Input: part model. Units: mm. Frame: model coordinates. Face numbers are marked on the shaded views. Give positions to 0.01 mm unless a question says otherwise; leave off trailing zeros. Write each loop counter-clockwise with the first axis right and the second up, starting at its lowest first coordinate (ties: lowest second). Pieces come first, ordered by that corner, then holes. Notation, with made-up numbers: (83, 37) - (91, 37) arc R35 cw to (91, 76) - close; hole circle Ø1 at (59, 31.25). An arc over 180 degrees is marked (long way). Use a Markdown table: item, result. Add a question column.
1. Section query D-D, the plane y = 10. Return loops of the section in (x, z), plus the area to 3 significant figures.
2. Section query C-C, the plane y = 3.75. Return loops of the section in (x, z), plus the area to 3 significant figures.
3. Section query B-B, the plane x = 70. Return loops of the section in (y, z).
4. Section query A-A, the plane z = 10.5. Return loops of the section in (x, y).
5. Mould query, pull axis Y, two halves, no side actions, for the marked faces 1, 2, 3 and 4. Classes: released by +Y, released by -Y, zero draft, split by the parting line, or undercut.
6. Pin query (flat end, axial travel): pin 1 (2 mm diameter, centred on y = -2, z = 11.5, fed in from -X). Return the tip coordinate at first contact, or that it passes through.
7. Material intervals for probe 1 along Y at (x, z) = (75, 12.5); probe 2 along X at (y, z) = (-2, 2.5); probe 3 along X at (y, z) = (4.25, 8.75), sorted ascending.
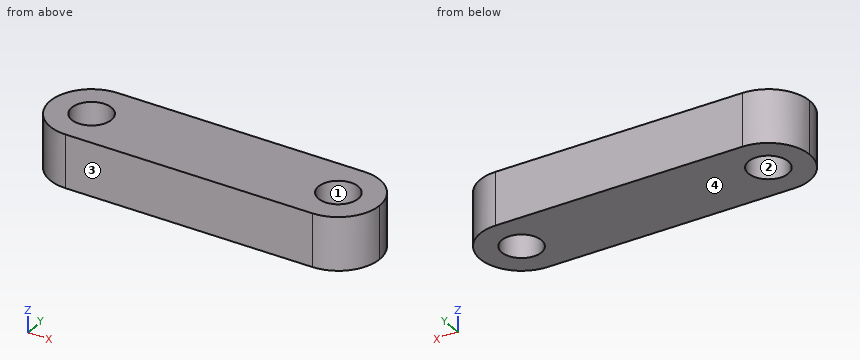
```python
from build123d import *

# Parameters (mm, degrees)
F0_R     = 6
F1_DEPTH = 16


# Not quite as in the source:
# - a feature names something its author has since deleted; it is built from what else it names


with BuildPart() as f1:
    # F0 (on Top) → F1 (new body)
    with BuildSketch(Plane.XY):
        with BuildLine():
            Line((75, 12.5), (0, 12.5))
            ThreePointArc((0, 12.5), (8.8388347648, 8.8388347648), (12.5, 0))
            ThreePointArc((12.5, 0), (8.8388347648, -8.8388347648), (0, -12.5))
            Line((0, -12.5), (75, -12.5))
            ThreePointArc((75, -12.5), (62.5, 0), (75, 12.5))
        make_face()
        with BuildLine():
            ThreePointArc((12.5, 0), (8.8388347648, 8.8388347648), (0, 12.5))
            ThreePointArc((0, 12.5), (-8.8388347648, 8.8388347648), (-12.5, 0))
            ThreePointArc((-12.5, 0), (-8.8388347648, -8.8388347648), (0, -12.5))
            ThreePointArc((0, -12.5), (8.8388347648, -8.8388347648), (12.5, 0))
        make_face()
        Circle(F0_R, mode=Mode.SUBTRACT)
        with BuildLine():
            ThreePointArc((87.5, 0), (83.8388347648, 8.8388347648), (75, 12.5))
            ThreePointArc((75, 12.5), (62.5, 0), (75, -12.5))
            ThreePointArc((75, -12.5), (83.8388347648, -8.8388347648), (87.5, 0))
        make_face()
        with Locations((75, 0)):
            Circle(F0_R, mode=Mode.SUBTRACT)
    extrude(amount=F1_DEPTH)


solid = f1.part
```
Result sheet:
| question | item | result |
|---|---|---|
| 1 | outline | (-7.5, 0) - (82.5, 0) - (82.5, 16) - (-7.5, 16) - close |
| 1 | area | 1,440 mm² |
| 2 | outline | (-11.92, 0) - (-4.68, 0) - (-4.68, 16) - (-11.92, 16) - close; (4.68, 0) - (70.32, 0) - (70.32, 16) - (4.68, 16) - close; (79.68, 0) - (86.92, 0) - (86.92, 16) - (79.68, 16) - close |
| 2 | area | 1,280 mm² |
| 3 | outline | (-12.5, 0) - (-3.32, 0) - (-3.32, 16) - (-12.5, 16) - close; (3.32, 0) - (12.5, 0) - (12.5, 16) - (3.32, 16) - close |
| 4 | outline | (0, -12.5) - (75, -12.5) arc R12.5 ccw to (75, 12.5) - (0, 12.5) arc R12.5 ccw to start; hole circle Ø12 at (0, 0); hole circle Ø12 at (75, 0) |
| 5 | face 1 | undercut |
| 5 | face 2 | undercut |
| 5 | face 3 | released by -Y |
| 5 | face 4 | zero draft |
| 6 | pin 1 | stops at x = -12.46 |
| 7 | probe 1 | y = -12.5 to -6, 6 to 12.5 |
| 7 | probe 2 | x = -12.34 to -5.66, 5.66 to 69.34, 80.66 to 87.34 |
| 7 | probe 3 | x = -11.76 to -4.24, 4.24 to 70.76, 79.24 to 86.76 |
